The model under review builds one solid part; all positions refer to its coordinate system, in mm. Round coordinates to 2 decimals unless told otherwise and drop trailing zeros. Loops run counter-clockwise (first coordinate to the right, second up) from the corner with the lowest first, then second, coordinate; pieces in that order, holes last. Notation, with made-up numbers: (5, 69.5) -> (19, 69.5) arc R28 cw to (19, 100.5) -> close; hole circle Ø8 at (-14.75, 78.25). An arc over 180 degrees is marked (long way). Use a Markdown table: item, result. Add a question column.
1) Consider section C-C on x = -29. Give the boundary of the cut face in (y, z).
2) Insertion check: pin 1 (6 mm diameter, centred on x = -110, y = -10, fed in from +Z); pin 2 (4.5 mm diameter, centred on x = -70, y = 10, fed in from -Z); pin 3 (1 mm diameter, centred on x = -137, z = 1.5, fed in from +Y); pin 4 (1.5 mm diameter, centred on y = 92, z = 2.5, fed in from -X). Each pin has a flat end and moves straight along its axis. Give the tip position at first contact, or say it passes through.
3) Wall thickness on probe 1 along Y at (x, z) = (-170, 4.5); probe 2 along X at (y, z) = (104, 5.5); probe 3 along Y at (x, z) = (45.5, 5.5): over which ranges is each line inside the solid? List them lowest first.
4) Consider section A-A on y = 88. Give the boundary of the cut face in (x, z).
5) Consider section B-B on z = 1.5. State how many separate pieces and enclosed holes the cut face has, plus the area to 3 significant figures.
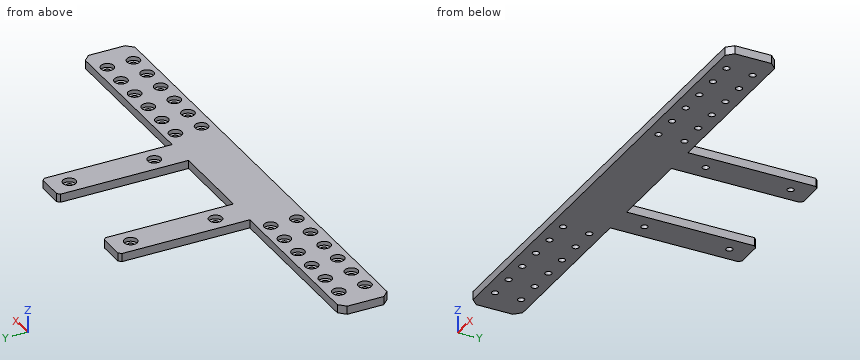
from build123d import *

# Parameters (mm, degrees)
SKETCH1_R           = 2.5
BOSS_EXTRUDE1_DEPTH = 6.4
SKETCH2_R           = 5
CUT_EXTRUDE1_DEPTH  = 3
CHAMFER1_SIZE       = 5
CHAMFER2_SIZE       = 2


with BuildPart() as part:
    # Sketch1 → Boss-Extrude1 (new body)
    with BuildSketch(Plane.XY):
        Polygon((190, -19.05), (-190, -19.05), (-190, 19.05), (-56.5, 19.05), (-56.5, 119.05), (-32.5, 119.05), (-32.5, 19.05), (33.5, 19.05), (33.5, 119.05), (57.5, 119.05), (57.5, 19.05), (190, 19.05), align=None)
        with Locations((-70, 10)):
            Circle(SKETCH1_R, mode=Mode.SUBTRACT)
        with Locations((-90, 10)):
            Circle(SKETCH1_R, mode=Mode.SUBTRACT)
        with Locations((-110, 10)):
            Circle(SKETCH1_R, mode=Mode.SUBTRACT)
        with Locations((-130, 10)):
            Circle(SKETCH1_R, mode=Mode.SUBTRACT)
        with Locations((-150, 10)):
            Circle(SKETCH1_R, mode=Mode.SUBTRACT)
        with Locations((-170, 10)):
            Circle(SKETCH1_R, mode=Mode.SUBTRACT)
        with Locations(Location((-70, -10, 0), (0, 0, 180))):
            Circle(SKETCH1_R, mode=Mode.SUBTRACT)
        with Locations(Location((-90, -10, 0), (0, 0, 180))):
            Circle(SKETCH1_R, mode=Mode.SUBTRACT)
        with Locations(Location((-110, -10, 0), (0, 0, 180))):
            Circle(SKETCH1_R, mode=Mode.SUBTRACT)
        with Locations(Location((-130, -10, 0), (0, 0, 180))):
            Circle(SKETCH1_R, mode=Mode.SUBTRACT)
        with Locations(Location((-150, -10, 0), (0, 0, 180))):
            Circle(SKETCH1_R, mode=Mode.SUBTRACT)
        with Locations(Location((-170, -10, 0), (0, 0, 180))):
            Circle(SKETCH1_R, mode=Mode.SUBTRACT)
        with Locations((170, -10)):
            Circle(SKETCH1_R, mode=Mode.SUBTRACT)
        with Locations((150, -10)):
            Circle(SKETCH1_R, mode=Mode.SUBTRACT)
        with Locations((130, -10)):
            Circle(SKETCH1_R, mode=Mode.SUBTRACT)
        with Locations((110, -10)):
            Circle(SKETCH1_R, mode=Mode.SUBTRACT)
        with Locations((90, -10)):
            Circle(SKETCH1_R, mode=Mode.SUBTRACT)
        with Locations((70, -10)):
            Circle(SKETCH1_R, mode=Mode.SUBTRACT)
        with Locations(Location((70, 10, 0), (0, 0, 180))):
            Circle(SKETCH1_R, mode=Mode.SUBTRACT)
        with Locations(Location((90, 10, 0), (0, 0, 180))):
            Circle(SKETCH1_R, mode=Mode.SUBTRACT)
        with Locations(Location((110, 10, 0), (0, 0, 180))):
            Circle(SKETCH1_R, mode=Mode.SUBTRACT)
        with Locations(Location((130, 10, 0), (0, 0, 180))):
            Circle(SKETCH1_R, mode=Mode.SUBTRACT)
        with Locations(Location((150, 10, 0), (0, 0, 180))):
            Circle(SKETCH1_R, mode=Mode.SUBTRACT)
        with Locations(Location((170, 10, 0), (0, 0, 180))):
            Circle(SKETCH1_R, mode=Mode.SUBTRACT)
        with Locations((-44.5, 39.05)):
            Circle(SKETCH1_R, mode=Mode.SUBTRACT)
        with Locations((-44.5, 104.05)):
            Circle(SKETCH1_R, mode=Mode.SUBTRACT)
        with Locations((45.5, 104.05)):
            Circle(SKETCH1_R, mode=Mode.SUBTRACT)
        with Locations((45.5, 39.05)):
            Circle(SKETCH1_R, mode=Mode.SUBTRACT)
    extrude(amount=BOSS_EXTRUDE1_DEPTH)

    # Sketch2 → Cut-Extrude1 (cut)
    with BuildSketch(Plane.XY.offset(6.4)):
        with Locations((-170, 10)):
            Circle(SKETCH2_R)
        with Locations((-150, 10)):
            Circle(SKETCH2_R)
        with Locations((-130, 10)):
            Circle(SKETCH2_R)
        with Locations((-110, 10)):
            Circle(SKETCH2_R)
        with Locations((-90, 10)):
            Circle(SKETCH2_R)
        with Locations((-70, 10)):
            Circle(SKETCH2_R)
        with Locations(Location((-70, -10, 0), (0, 0, 180))):
            Circle(SKETCH2_R)
        with Locations(Location((-90, -10, 0), (0, 0, 180))):
            Circle(SKETCH2_R)
        with Locations(Location((-110, -10, 0), (0, 0, 180))):
            Circle(SKETCH2_R)
        with Locations(Location((-130, -10, 0), (0, 0, 180))):
            Circle(SKETCH2_R)
        with Locations(Location((-150, -10, 0), (0, 0, 180))):
            Circle(SKETCH2_R)
        with Locations(Location((-170, -10, 0), (0, 0, 180))):
            Circle(SKETCH2_R)
        with Locations((170, -10)):
            Circle(SKETCH2_R)
        with Locations((150, -10)):
            Circle(SKETCH2_R)
        with Locations((130, -10)):
            Circle(SKETCH2_R)
        with Locations((110, -10)):
            Circle(SKETCH2_R)
        with Locations((90, -10)):
            Circle(SKETCH2_R)
        with Locations((70, -10)):
            Circle(SKETCH2_R)
        with Locations(Location((70, 10, 0), (0, 0, 180))):
            Circle(SKETCH2_R)
        with Locations(Location((90, 10, 0), (0, 0, 180))):
            Circle(SKETCH2_R)
        with Locations(Location((110, 10, 0), (0, 0, 180))):
            Circle(SKETCH2_R)
        with Locations(Location((130, 10, 0), (0, 0, 180))):
            Circle(SKETCH2_R)
        with Locations(Location((150, 10, 0), (0, 0, 180))):
            Circle(SKETCH2_R)
        with Locations(Location((170, 10, 0), (0, 0, 180))):
            Circle(SKETCH2_R)
        with Locations((-44.5, 104.05)):
            Circle(SKETCH2_R)
        with Locations((-44.5, 39.05)):
            Circle(SKETCH2_R)
        with Locations((45.5, 39.05)):
            Circle(SKETCH2_R)
        with Locations((45.5, 104.05)):
            Circle(SKETCH2_R)
    extrude(amount=-CUT_EXTRUDE1_DEPTH, mode=Mode.SUBTRACT)

    # Chamfer1
    chamfer1_edges = [part.edges().sort_by_distance(p)[0] for p in [
        (190, 19.05, 3.2),
        (190, -19.05, 3.2),
        (-190, -19.05, 3.2),
        (-190, 19.05, 3.2),
    ]]
    chamfer(chamfer1_edges, length=CHAMFER1_SIZE)

    # Chamfer2
    chamfer2_edges = [part.edges().sort_by_distance(p)[0] for p in [
        (-56.5, 119.05, 3.2),
        (-32.5, 119.05, 3.2),
        (33.5, 119.05, 3.2),
        (57.5, 119.05, 3.2),
    ]]
    chamfer(chamfer2_edges, length=CHAMFER2_SIZE)


solid = part.part
Result set:
| question | item | result |
|---|---|---|
| 1 | outline | (-19.05, 0) -> (19.05, 0) -> (19.05, 6.4) -> (-19.05, 6.4) -> close |
| 2 | pin 1 | z = 3.4 |
| 2 | pin 2 | through |
| 2 | pin 3 | y = 19.05 |
| 2 | pin 4 | x = -56.5 |
| 3 | probe 1 | -19.05 to -15, -5 to 5, 15 to 19.05 |
| 3 | probe 2 | -56.5 to -49.5, -39.5 to -32.5, 33.5 to 40.5, 50.5 to 57.5 |
| 3 | probe 3 | -19.05 to 34.05, 44.05 to 99.05, 109.05 to 119.05 |
| 4 | outline | (-56.5, 0) -> (-32.5, 0) -> (-32.5, 6.4) -> (-56.5, 6.4) -> close; (33.5, 0) -> (57.5, 0) -> (57.5, 6.4) -> (33.5, 6.4) -> close |
| 5 | separate pieces | 1 |
| 5 | enclosed holes | 28 |
| 5 | area | 18,700 mm2 |
